Job drawing, mm, ordinate dimensions from the low corner. One solid piece. Round coordinates to 2 decimals unless told otherwise and drop trailing zeros. Loops run counter-clockwise (first coordinate to the right, second up) from the corner with the lowest first, then second, coordinate; pieces in that order, holes last. Notation, with made-up numbers: M 69,88 L 85,88 A27 cw 85,108 Z; hole C 0.25,21 d3. An arc over 180 degrees is marked long. One line per item, written item: value.
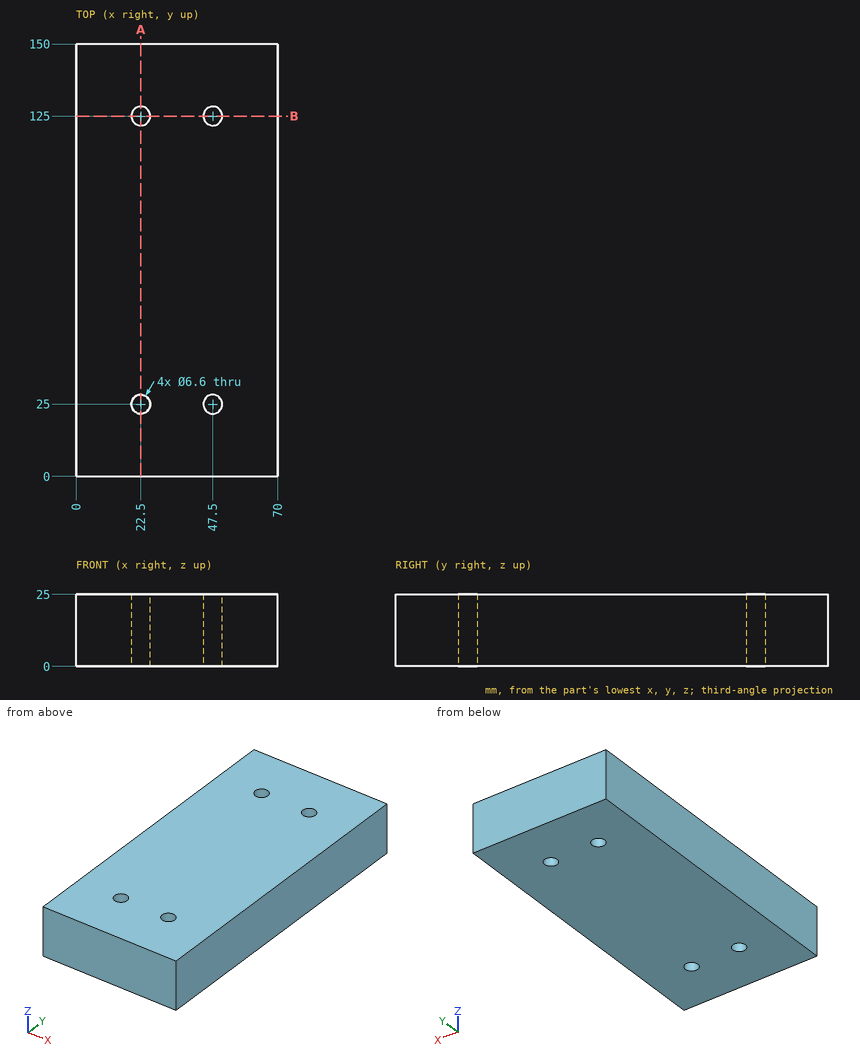
Item 1: Slice it at B-B, the plane y = 125. Give the cut face in (x, z), and give its area (3 significant figures).
Check values:
outline: M 0,0 L 19.2,0 L 19.2,25 L 0,25 Z; M 25.8,0 L 44.2,0 L 44.2,25 L 25.8,25 Z; M 50.8,0 L 70,0 L 70,25 L 50.8,25 Z
area: 1,420 mm2
Item 2: Slice it at A-A, the plane x = 22.5. Give the cut face in (y, z).
Check values:
outline: M 0,0 L 21.7,0 L 21.7,25 L 0,25 Z; M 28.3,0 L 121.7,0 L 121.7,25 L 28.3,25 Z; M 128.3,0 L 150,0 L 150,25 L 128.3,25 Z
Item 3: Wall check: line 1 along Y through (x, z) = (47.5, 13.75); line 2 along X through (y, z) = (23, 15.5). Give the ranges that are in metal, low to high.
Check values:
line 1: y = 0 to 21.7, 28.3 to 121.7, 128.3 to 150
line 2: x = 0 to 19.88, 25.12 to 44.88, 50.12 to 70
